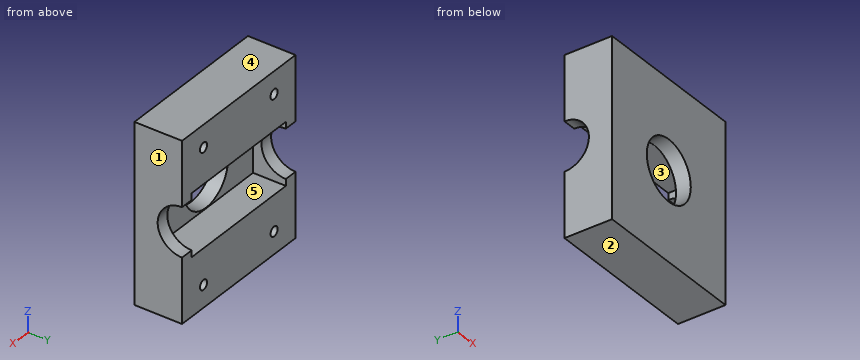
from build123d import *

# Parameters (mm, degrees)
SKETCH1_W             = 52.9
SKETCH1_H             = 30
SKETCH1_R             = 10.25
BOSS_EXTRUDE1_DEPTH   = 5
SKETCH3_W             = 52.9
SKETCH3_H             = 30
SKETCH3_W_2           = 43.9
SKETCH3_H_2           = 21
BOSS_EXTRUDE2_DEPTH   = 11.1
SKETCH4_R             = 8.25
CUT_EXTRUDE1_DEPTH    = 53.9
SKETCH5_W             = 52.9
SKETCH5_H             = 5
BOSS_EXTRUDE3_DEPTH   = 15
SKETCH6_W             = 52.9
SKETCH6_H             = 5
BOSS_EXTRUDE4_DEPTH   = 15
SKETCH7_W             = 52.9
SKETCH7_H             = 15
BOSS_EXTRUDE5_DEPTH   = 11.1
M4_TAPPED_HOLE1_D     = 3.3
M4_TAPPED_HOLE1_DEPTH = 9.108579979
M4_TAPPED_HOLE1_TIP   = 0.991420021


with BuildPart() as part:
    # Sketch1 → Boss-Extrude1 (new body)
    with BuildSketch(Plane(origin=(0, 0, 0), x_dir=(1, 0, 0), z_dir=(0, 1, 0))):
        Rectangle(SKETCH1_W, SKETCH1_H)
        Circle(SKETCH1_R, mode=Mode.SUBTRACT)
    extrude(amount=BOSS_EXTRUDE1_DEPTH)

    # Sketch3 → Boss-Extrude2 (add)
    with BuildSketch(Plane(origin=(0, 5, 0), x_dir=(1, 0, 0), z_dir=(0, 1, 0))):
        Rectangle(SKETCH3_W, SKETCH3_H)
        Rectangle(SKETCH3_W_2, SKETCH3_H_2, mode=Mode.SUBTRACT)
    extrude(amount=BOSS_EXTRUDE2_DEPTH)

    # Sketch4 → Cut-Extrude1 (cut, through all)
    with BuildSketch(Plane(origin=(26.45, 0, 0), x_dir=(0, 0, -1), z_dir=(1, 0, 0))):
        with Locations((0, 16.1)):
            Circle(SKETCH4_R)
    extrude(amount=-CUT_EXTRUDE1_DEPTH, mode=Mode.SUBTRACT)

    # Sketch5 → Boss-Extrude3 (add)
    with BuildSketch(Plane.XY.offset(15)):
        with Locations((0, 13.6)):
            Rectangle(SKETCH5_W, SKETCH5_H)
    extrude(amount=BOSS_EXTRUDE3_DEPTH)

    # Sketch6 → Boss-Extrude4 (add)
    with BuildSketch(Plane(origin=(0, 0, -15), x_dir=(-1, 0, 0), z_dir=(0, 0, -1))):
        with Locations((0, 13.6)):
            Rectangle(SKETCH6_W, SKETCH6_H)
    extrude(amount=BOSS_EXTRUDE4_DEPTH)

    # Sketch7 → Boss-Extrude5 (add)
    with BuildSketch(Plane.XZ.offset(-11.1)):
        with Locations((0, 22.5)):
            Rectangle(SKETCH7_W, SKETCH7_H)
        with Locations((0, -22.5)):
            Rectangle(SKETCH7_W, SKETCH7_H)
    extrude(amount=BOSS_EXTRUDE5_DEPTH)

    # M4 Tapped Hole1
    with Locations(Plane(origin=(0, 16.1, 0), x_dir=(1, 0, 0), z_dir=(0, 1, 0))):
        with Locations((-16.45, -22.5), (16.45, -22.5), (16.45, 22.5), (-16.45, 22.5)):
            Hole(M4_TAPPED_HOLE1_D / 2, depth=M4_TAPPED_HOLE1_DEPTH)
            with Locations((0, 0, -(M4_TAPPED_HOLE1_DEPTH + M4_TAPPED_HOLE1_TIP / 2))):  # 118° drill point
                Cone(0, M4_TAPPED_HOLE1_D / 2, M4_TAPPED_HOLE1_TIP, mode=Mode.SUBTRACT)


solid = part.part
For this review, take the finished solid that the model builds, in its own axes (mm). Face numbers are marked on the shaded views. A direction names the side the tool comes from. Round coordinates to 2 decimals unless told otherwise and drop trailing zeros. Write each loop counter-clockwise with the first axis right and the second up, starting at its lowest first coordinate (ties: lowest second). Pieces come first, ordered by that corner, then holes. Notation, with made-up numbers: (57.25, -4) -> (107.25, -4) arc R21 ccw to (107.25, 6) -> close; hole circle Ø7 at (32.5, 54). An arc over 180 degrees is marked (long way). Put each result on its own line as item: value.
Q1. Clearance check with flat-ended pins moving along their axes: pin 1 Ø2 at (y, z) = (11, -4.5) entering from -X; pin 2 Ø2 at (x, z) = (16.45, 22.5) entering from +Y; pin 3 Ø17 at (x, z) = (-8.5, -1.5) entering from +Y. State where each tip first meets the part, or that it passes through.
Determined:
pin 1: passes through
pin 2: stops at y = 6.6
pin 3: stops at y = 5
Q2. Consider section A-A on z = 0. State the section outline as (x, y) points.
Determined:
outline: (-26.45, 0) -> (-10.25, 0) -> (-10.25, 5) -> (-21.95, 5) -> (-21.95, 7.85) -> (-26.45, 7.85) -> close; (10.25, 0) -> (26.45, 0) -> (26.45, 7.85) -> (21.95, 7.85) -> (21.95, 5) -> (10.25, 5) -> close
Q3. Machinability: for the marked faces 4 and 5, which of the approach directions +Z, -Z, +X, -X, +Y, -Y give a long, thin tool a straight path to every point of the face, cutting with its end or side? Answer none if there is none.
Determined:
face 4: +Z, +X, -X, +Y, -Y
face 5: +Y
Q4. Consider section B-B on y = 11. State the section outline as (x, z) points, and give its area (3 significant figures).
Determined:
outline: (-26.45, -30) -> (26.45, -30) -> (26.45, -6.48) -> (21.95, -6.48) -> (21.95, -10.5) -> (-21.95, -10.5) -> (-21.95, -6.48) -> (-26.45, -6.48) -> close; (-26.45, 6.48) -> (-21.95, 6.48) -> (-21.95, 10.5) -> (21.95, 10.5) -> (21.95, 6.48) -> (26.45, 6.48) -> (26.45, 30) -> (-26.45, 30) -> close; hole circle Ø3.3 at (-16.45, -22.5); hole circle Ø3.3 at (-16.45, 22.5); hole circle Ø3.3 at (16.45, -22.5); hole circle Ø3.3 at (16.45, 22.5)
area: 2,100 mm^2
Q5. To check wall thickness, follow L1, parallel to Z at x = -16.45, y = 12; L2, parallel to X at y = 9.5, z = 22.5; L3, parallel to Z at x = 14, y = 11.75. State the ranges of each line that lie inside material, in increasing order. Write a range as [from, to].
Determined:
L1: z = [-30, -24.15], [-20.85, -10.5], [10.5, 20.85], [24.15, 30]
L2: x = [-26.45, -18.1], [-14.8, 14.8], [18.1, 26.45]
L3: z = [-30, -10.5], [10.5, 30]
Q6. Consider section D-D on x = -21. State the section outline as (y, z) points, and give its area (3 significant figures).
Determined:
outline: (0, -30) -> (16.1, -30) -> (16.1, -10.5) -> (5, -10.5) -> (5, 10.5) -> (16.1, 10.5) -> (16.1, 30) -> (0, 30) -> close
area: 733 mm^2
Q7. The part is to be moulded in two halves that separate along Z. For the marked faces 1, 2 and 3, say which applies: released by +Z, released by -Z, zero draft, split by the parting line, or undercut.
Determined:
face 1: zero draft
face 2: released by -Z
face 3: undercut
Q8. Consider section C-C on x = 0. State the section outline as (y, z) points, and give its area (3 significant figures).
Determined:
outline: (0, -30) -> (16.1, -30) -> (16.1, -10.5) -> (5, -10.5) -> (5, -10.25) -> (0, -10.25) -> close; (0, 10.25) -> (5, 10.25) -> (5, 10.5) -> (16.1, 10.5) -> (16.1, 30) -> (0, 30) -> close
area: 630 mm^2
